Geometry check sheet. Reference: the model listing, model coordinates, mm. Face numbers are marked on the shaded views. A direction names the side the tool comes from. Give positions to 0.01 mm unless a question says otherwise; leave off trailing zeros. Loops run counter-clockwise (first coordinate to the right, second up) from the corner with the lowest first, then second, coordinate; pieces in that order, holes last. Notation, with made-up numbers: (63.25, 25) - (73.25, 25) arc R15 cw to (73.25, 33) - close; hole circle Ø4 at (64.25, 41.5). An arc over 180 degrees is marked (long way). Use a Markdown table: item, result. Add a question column.
1. Cross-section at C-C on y = 23. Enter the section's corners in (x, z), and give its area (3 significant figures).
2. Cross-section at A-A on x = -10. Enter the section's corners in (y, z).
3. Material ranges on L1, parallel to Y at x = 2, z = 8; L2, parallel to Z at x = -8.5, y = 45; L3, parallel to X at y = 26, z = 0.25, recorded low to high.
4. Depth check by flat-ended pin: P1, Ø0.9, axis at y = 21.5, z = 3, coming from the +X side; P2, Ø1.2, axis at y = 54.5, z = 11, coming from the +X side; P3, Ø10, axis at y = 27.5, z = -6, coming from the -X side. Enter the tip coordinate at first touch or a pass-through.
5. Cross-section at D-D on x = 5.5. Enter the section's corners in (y, z).
6. Set-up check for the marked faces 1 and 2: record each of +Z, -Z, +X, -X, +Y, -Y from which the full face is reachable in a straight line by a thin tool's end or side.
7. Draft check along Z on the marked faces 3, 4, 5 and 6. Enter one of: pulls with the +Z half, pulls with the -Z half, needs draft (parallel to the pull), parting line crosses it, or undercut.
from build123d import *

# Parameters (mm, degrees)
BOSS_EXTRUDE1_DEPTH = 53
BOSS_EXTRUDE2_DEPTH = 2.5
SKETCH3_W           = 19
SKETCH3_H           = 2.5
BOSS_EXTRUDE3_DEPTH = 4
SKETCH4_W           = 9.555688256
SKETCH4_H           = 10
CUT_EXTRUDE1_DEPTH  = 10
FILLET2_R           = 4
FILLET3_R           = 4


with BuildPart() as part:
    # Sketch1 → Boss-Extrude1 (new body)
    with BuildSketch(Plane(origin=(0, 0, 0), x_dir=(1, 0, 0), z_dir=(0, 1, 0))):
        with BuildLine():
            Line((-6.997142274, 12.7), (-11.313185358, 12.7))
            Line((-11.313185358, 12.7), (-11.695935453, 12.337142857))
            ThreePointArc((-11.695935453, 12.337142857), (-17, 0), (-11.695935453, -12.337142857))
            Line((-11.695935453, -12.337142857), (-11.313185358, -12.7))
            Line((-11.313185358, -12.7), (-6.997142274, -12.7))
            ThreePointArc((-6.997142274, -12.7), (-14.5, 0), (-6.997142274, 12.7))
        make_face()
    extrude(amount=BOSS_EXTRUDE1_DEPTH)

    # Sketch2 → Boss-Extrude2 (add)
    with BuildSketch(Plane(origin=(0, 53, 0), x_dir=(1, 0, 0), z_dir=(0, 1, 0))):
        with BuildLine():
            Line((10.046814642, 12.7), (10.046814642, -12.7))
            Line((10.046814642, -12.7), (-11.313185358, -12.7))
            ThreePointArc((-11.313185358, -12.7), (-17, 0), (-11.313185358, 12.7))
            Line((-11.313185358, 12.7), (10.046814642, 12.7))
        make_face()
    extrude(amount=BOSS_EXTRUDE2_DEPTH)

    # Sketch3 → Boss-Extrude3 (add)
    with BuildSketch(Plane(origin=(10.046814642, 0, 0), x_dir=(0, 0, -1), z_dir=(1, 0, 0))):
        with Locations((0.5, 54.25)):
            Rectangle(SKETCH3_W, SKETCH3_H)
    extrude(amount=BOSS_EXTRUDE3_DEPTH)

    # Sketch4 → Cut-Extrude1 (cut)
    with BuildSketch(Plane.XY.offset(12.7)):
        with Locations((-11.774986402, 23)):
            Rectangle(SKETCH4_W, SKETCH4_H)
    extrude(amount=-CUT_EXTRUDE1_DEPTH, mode=Mode.SUBTRACT)

    # Fillet2
    fillet2_edges = [part.edges().sort_by_distance(p)[0] for p in [
        (14.046814642, 54.25, -10),
        (14.046814642, 54.25, 9),
    ]]
    fillet(fillet2_edges, radius=FILLET2_R - 0.0001)  # a hair under: the kernel refuses the full size

    # Fillet3
    fillet3_edges = [part.edges().sort_by_distance(p)[0] for p in [
        (-15.399616792, 18, 2.7),
        (-15.399616792, 28, 2.7),
    ]]
    fillet(fillet3_edges, radius=FILLET3_R)


solid = part.part
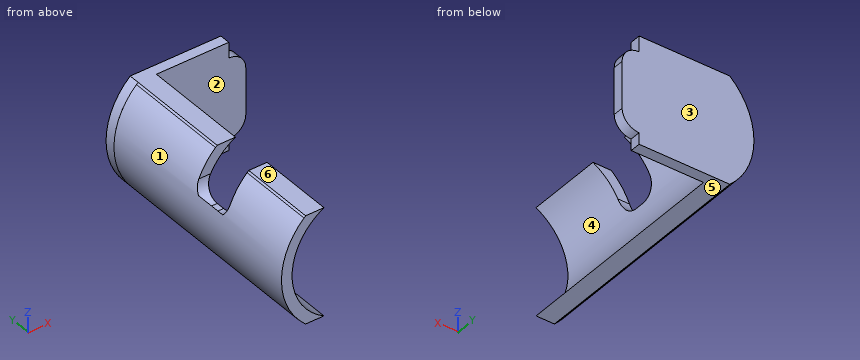
Values found:
| question | item | result |
|---|---|---|
| 1 | outline | (-16.55, 2.7) - (-16.55, 3.87) arc R17 ccw to (-11.7, -12.34) - (-11.31, -12.7) - (-7, -12.7) arc R14.5 cw to (-14.25, 2.7) - close |
| 1 | area | 44.0 mm2 |
| 2 | outline | (0, -12.7) - (55.5, -12.7) - (55.5, 12.7) - (28, 12.7) - (28, 10.5) - (53, 10.5) - (53, -10.5) - (0, -10.5) - close; (0, 10.5) - (18, 10.5) - (18, 12.7) - (0, 12.7) - close |
| 3 | L1 | y = 53 to 55.5 |
| 3 | L2 | z = -12.7 to -11.75, 11.75 to 12.7 |
| 3 | L3 | x = -17 to -14.5 |
| 4 | P1 | stops at x = -14.23 |
| 4 | P2 | stops at x = 10.05 |
| 4 | P3 | stops at x = -16.97 |
| 5 | outline | (53, -12.7) - (55.5, -12.7) - (55.5, 12.7) - (53, 12.7) - close |
| 6 | face 1 | -X, +Y, -Y |
| 6 | face 2 | +X, -Y |
| 7 | face 3 | needs draft |
| 7 | face 4 | undercut |
| 7 | face 5 | pulls with the -Z half |
| 7 | face 6 | pulls with the +Z half |
